from build123d import *

# Parameters (mm, degrees)
SKETCH2_W           = 67.8
SKETCH2_H           = 67.8
BOSS_EXTRUDE1_DEPTH = 35
FILLET1_R           = 3
SKETCH3_R           = 3.65
CUT_EXTRUDE1_DEPTH  = 38.6
SKETCH4_R           = 3.65
CUT_EXTRUDE2_DEPTH  = 38.6
SKETCH5_R           = 3.65
CUT_EXTRUDE3_DEPTH  = 38.6
SKETCH6_R           = 3.65
CUT_EXTRUDE4_DEPTH  = 38.6
SKETCH7_R           = 8
BOSS_EXTRUDE2_DEPTH = 5
SKETCH8_R           = 2.675
CUT_EXTRUDE5_DEPTH  = 17.9
FILLET2_R           = 1
BOSS_EXTRUDE3_DEPTH = 67.8
FILLET3_R           = 2


with BuildPart() as part:
    # Sketch2 → Boss-Extrude1 (new, symmetric)
    with BuildSketch(Plane.XY):
        Rectangle(SKETCH2_W, SKETCH2_H)
        Polygon((3.2, 16), (6.2, 16), (6.2, 31.9), (31.9, 31.9), (31.9, 6.2), (16, 6.2), (16, 3.2), (31.9, 3.2), (31.9, -3.2), (16, -3.2), (16, -6.2), (31.9, -6.2), (31.9, -31.9), (6.2, -31.9), (6.2, -16), (3.2, -16), (3.2, -31.9), (-3.2, -31.9), (-3.2, -16), (-6.2, -16), (-6.2, -31.9), (-31.9, -31.9), (-31.9, -6.2), (-16, -6.2), (-16, -3.2), (-31.9, -3.2), (-31.9, 3.2), (-16, 3.2), (-16, 6.2), (-31.9, 6.2), (-31.9, 31.9), (-6.2, 31.9), (-6.2, 16), (-3.2, 16), (-3.2, 31.9), (3.2, 31.9), align=None, mode=Mode.SUBTRACT)
    extrude(amount=BOSS_EXTRUDE1_DEPTH, both=True)

    # Fillet1
    fillet1_edges = [part.edges().sort_by_distance(p)[0] for p in [
        (-31.9, -6.2, 0),
        (-31.9, -31.9, 0),
        (-6.2, -31.9, 0),
        (6.2, -31.9, 0),
        (31.9, -31.9, 0),
        (31.9, -6.2, 0),
        (31.9, 6.2, 0),
        (31.9, 31.9, 0),
        (6.2, 31.9, 0),
        (-6.2, 31.9, 0),
        (-31.9, 31.9, 0),
        (-31.9, 6.2, 0),
    ]]
    fillet(fillet1_edges, radius=FILLET1_R)

    # Sketch3 → Cut-Extrude1 (cut)
    with BuildSketch(Plane(origin=(0, 33.9, 0), x_dir=(1, 0, 0), z_dir=(0, 1, 0))):
        with Locations(Location((-21.7, -22.5, 0), (0, 0, 270))):
            Circle(SKETCH3_R)
        with Locations(Location((-21.7, 22.5, 0), (0, 0, 270))):
            Circle(SKETCH3_R)
    extrude(amount=-CUT_EXTRUDE1_DEPTH, mode=Mode.SUBTRACT)

    # Sketch4 → Cut-Extrude2 (cut)
    with BuildSketch(Plane(origin=(33.9, 0, 0), x_dir=(0, 0, -1), z_dir=(1, 0, 0))):
        with Locations((22.5, 21.7)):
            Circle(SKETCH4_R)
        with Locations((-22.5, 21.7)):
            Circle(SKETCH4_R)
    extrude(amount=-CUT_EXTRUDE2_DEPTH, mode=Mode.SUBTRACT)

    # Sketch5 → Cut-Extrude3 (cut)
    with BuildSketch(Plane.XZ.offset(33.9)):
        with Locations((21.7, -22.5)):
            Circle(SKETCH5_R)
        with Locations((21.7, 22.5)):
            Circle(SKETCH5_R)
    extrude(amount=-CUT_EXTRUDE3_DEPTH, mode=Mode.SUBTRACT)

    # Sketch6 → Cut-Extrude4 (cut)
    with BuildSketch(Plane.ZY.offset(33.9)):
        with Locations(Location((-22.5, -21.7, 0), (0, 0, 270))):
            Circle(SKETCH6_R)
        with Locations(Location((22.5, -21.7, 0), (0, 0, 270))):
            Circle(SKETCH6_R)
    extrude(amount=-CUT_EXTRUDE4_DEPTH, mode=Mode.SUBTRACT)

    # Sketch7 → Boss-Extrude2 (add)
    with BuildSketch(Plane(origin=(33.9, 0, 0), x_dir=(0, 0, -1), z_dir=(1, 0, 0))):
        with Locations(Location((0, 0, 0), (0, 0, 180))):
            Circle(SKETCH7_R)
        Polygon((2.3375, 4.048668763), (-2.3375, 4.048668763), (-4.675, 0), (-2.3375, -4.048668763), (2.3375, -4.048668763), (4.675, 0), align=None, mode=Mode.SUBTRACT)
    extrude(amount=BOSS_EXTRUDE2_DEPTH)

    # Sketch8 → Cut-Extrude5 (cut)
    with BuildSketch(Plane(origin=(33.9, 0, 0), x_dir=(0, 0, -1), z_dir=(1, 0, 0))):
        Circle(SKETCH8_R)
    extrude(amount=-CUT_EXTRUDE5_DEPTH, mode=Mode.SUBTRACT)

    # Fillet2
    fillet2_edges = [part.edges().sort_by_distance(p)[0] for p in [
        (33.9, 0, -8),
    ]]
    fillet(fillet2_edges, radius=FILLET2_R)

    # Sketch9 → Boss-Extrude3 (add)
    with BuildSketch(Plane(origin=(33.9, 0, 0), x_dir=(0, 0, -1), z_dir=(1, 0, 0))):
        Polygon((5.15, 33.9), (5.15, 43.9), (8.35, 43.9), (8.35, 31.9), (-8.35, 31.9), (-8.35, 33.9), (-10.35, 33.9), (-10.35, 43.9), (-5.15, 43.9), (-5.15, 40.85), (-7.15, 40.85), (-7.15, 36.95), (-5.15, 36.95), (-5.15, 33.9), align=None)
    extrude(amount=-BOSS_EXTRUDE3_DEPTH)

    # Fillet3
    fillet3_edges = [part.edges().sort_by_distance(p)[0] for p in [
        (0, 33.9, -8.35),
        (0, 33.9, 10.35),
    ]]
    fillet(fillet3_edges, radius=FILLET3_R)


solid = part.part
CAD build for the part. Positions are in the model's coordinates, mm. A direction names the side the tool comes from. Coordinates: 2 decimals unless noted, no trailing zeros. Loops run counter-clockwise (first coordinate to the right, second up) from the corner with the lowest first, then second, coordinate; pieces in that order, holes last. Notation, with made-up numbers: (23.5, -33.5) - (70.5, -33.5) arc R29 cw to (70.5, -0.5) - close; hole circle Ø4 at (-9.75, -13.75). An arc over 180 degrees is marked (long way). Use one line per item in the form item = value. Start each with the question number.
1) Band-saw the part on B-B (z = 22.5). State how many separate pieces and enclosed holes the cut face has, and give its area (3 significant figures).
2) Flat gauge pins, fed straight in: pin 1 (3.5 mm diameter, centred on x = -20.5, z = -22, fed in from +Y); pin 2 (3 mm diameter, centred on y = -16, z = 19, fed in from +X); pin 3 (6.5 mm diameter, centred on x = 1.5, y = 40.5, fed in from -Z). Where does each tip first touch, or does it go through?
3) Tool access for faces 1 (the face through (-19.23, 4.72, 19.81)), 2 (the face through (0, 40, 10.35)), 3 (the face through (32.914, 21.86, 26.146)), 4 (the face through (-31.9, 19, 0)): list every direction of +Z, -Z, +X, -X, +Y, -Y with a clear straight run to the whole face (end or side of a thin tool).
4) Band-saw the part on A-A (x = 12.5). Give the cut face in (y, z), and give its area (3 significant figures).
5) Drill centre lines: L1, parallel to Y at x = 25.5, z = -22.5; L2, parallel to X at y = -10.5, z = 32. Where is each one in solid material? Low to high. Write a range as from..to.
6) Two-plate mould, pull along X, no slides. Class faces 5 (the face through (16, 5, 0)), 6 (the face through (0, 33.9, 24)), 7 (the face through (-4.7, 22, 23)), 8 (the face through (-33.9, 6, 0)): +X half, -X half, draft (parallel to the pull), parting line (faces both ways), or undercut.
Check values:
q1.separate_pieces = 8
q1.enclosed_holes = 0
q1.area = 741 mm2
q2.pin_1 = -4.7
q2.pin_2 = 33.9
q2.pin_3 = -8.35
q3.face_1 = +Y
q3.face_2 = +Z, +X, -X, +Y
q3.face_3 = +X
q3.face_4 = +Z, -Z
q4.outline = (-33.9, -35) - (-31.9, -35) - (-31.9, 35) - (-33.9, 35) - close; (31.9, -35) - (33.9, -35) - (33.9, -10.35) arc R2 cw to (35.9, -8.35) - (43.9, -8.35) - (43.9, -5.15) - (33.9, -5.15) - (33.9, 5.15) - (36.95, 5.15) - (36.95, 7.15) - (40.85, 7.15) - (40.85, 5.15) - (43.9, 5.15) - (43.9, 10.35) - (35.9, 10.35) arc R2 cw to (33.9, 12.35) - (33.9, 35) - (31.9, 35) - close
q4.area = 358 mm2
q5.L1 = -33.9..-31.9, -6.2..-3.2, 3.2..6.2, 31.9..33.9
q5.L2 = -33.9..-31.9, 31.9..33.9
q6.face_5 = undercut
q6.face_6 = draft
q6.face_7 = +X half
q6.face_8 = -X half
